Autodesk Inventor part; units mm, degrees
ref_plane "YZ Plane" through (0, 0, 0) normal (1, 0, 0) x (0, 1, 0)
ref_plane "XZ Plane" through (0, 0, 0) normal (0, 1, 0) x (-1, 0, 0)
ref_plane "XY Plane" through (0, 0, 0) normal (0, 0, 1) x (1, 0, 0)
sketch "スケッチ1" plane through (0, 0, 0) normal (0, 0, 1) x (1, 0, 0)
  circle A0 centre (59.9649, 0.0002) radius 1.5
  circle A1 centre (9.9649, 0.0002) radius 2
  circle A2 centre (-5.0351, 0.0002) radius 2
  circle A3 centre (50.4166, -7.2682) radius 1.5
  circle A4 centre (7.9649, -9.9998) radius 1.5
  arc A5 (-5.2274, 4.9965) -> (-7.9614, -4.054) centre (-5.0351, 0.0002) ccw
  line L0 (-7.9614, -4.054) -> (5.3313, -13.6486)
  arc A6 (5.3313, -13.6486) -> (7.4492, -14.4702) centre (7.9649, -9.9998) ccw
  line L1 (7.4492, -14.4702) -> (59.4492, -20.4691)
  arc A7 (59.4492, -20.4691) -> (64.3851, -16.8426) centre (59.9649, -15.9988) ccw
  line L2 (64.3851, -16.8426) -> (67.3319, -1.4061)
  arc A8 (67.3319, -1.4061) -> (59.6765, 7.4946) centre (59.9649, 0.0002) ccw
  line L3 (59.6765, 7.4946) -> (-5.2274, 4.9965)
  circle A9 centre (59.9649, 0.0002) radius 3
  circle A10 centre (50.4166, -7.2682) radius 3
  circle A11 centre (7.9649, -9.9998) radius 3
  circle A12 centre (36.9539, 0.0002) radius 1.5
  circle A13 centre (36.9539, 0.0002) radius 3
  arc A14 (36.6995, 6.6103) -> (33.5984, -5.7005) centre (36.9539, 0.0002) ccw
  line L4 (7.4492, -14.4702) -> (59.4492, -20.4691)
  arc A15 (57.6822, -19.8768) -> (59.4492, -20.4691) centre (59.9649, -15.9988) ccw
  line L5 (33.5984, -5.7005) -> (57.6822, -19.8768)
  line L6 (59.6765, 7.4946) -> (-5.2274, 4.9965)
  point P0 (0, 0)
  point P1 (0, 0)
  dimension "d0" = 6
  dimension "d1" = 6
  dimension "d2" = 6
  dimension "d3" = 6
extrude "押し出し1" add sketch "スケッチ1" along normal blind 3 contours L3 A8 L2 A7 A15 L5 A14 | A9 | A10 | A13
extrude "押し出し2" cut sketch "スケッチ1" along normal blind 1 contours A9 | A10 | A13
sketch "スケッチ2" plane through (0, 0, 0) normal (0, 0, -1) x (-1, 0, 0)
  circle A0 centre (-59.9649, 0.0002) radius 3
  circle A1 centre (-50.4166, -7.2682) radius 3
  circle A2 centre (-36.9539, 0.0002) radius 3
  line L0 (-59.6765, 7.4946) -> (-36.6995, 6.6103)
  arc A3 (-59.6765, 7.4946) -> (-67.3319, -1.4061) centre (-59.9649, 0.0002) ccw
  line L1 (-64.3851, -16.8426) -> (-67.3319, -1.4061)
  arc A4 (-64.3851, -16.8426) -> (-57.6822, -19.8768) centre (-59.9649, -15.9988) ccw
  line L2 (-33.5984, -5.7005) -> (-57.6822, -19.8768)
  arc A5 (-33.5984, -5.7005) -> (-36.6995, 6.6103) centre (-36.9539, 0.0002) ccw
  circle A6 centre (-59.9649, 0.0002) radius 1.5
  circle A7 centre (-50.4166, -7.2682) radius 1.5
  circle A8 centre (-36.9539, 0.0002) radius 1.5
  point P0 (0, 0)
properties part number "ツイン抑え" material "ポリカーボネート、クリア"
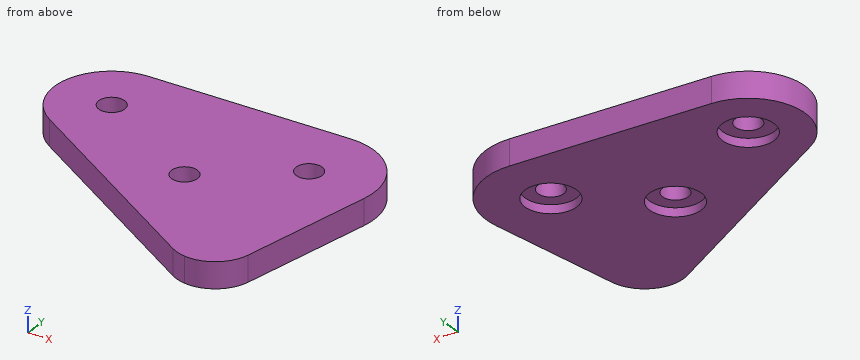
The model under review builds one solid part; all positions refer to its coordinate system, in mm. Coordinates: 2 decimals unless noted, no trailing zeros. Order: outer loops, then holes, each group sorted by start corner. A loop starts at its lowest first (then second) coordinate and runs counter-clockwise, first axis right, second up. Notation, with made-up numbers: M 5,71.25 L 10,71.25 A26 ccw 10,107.25 Z; hole C 64.5,28.25 d4. An arc over 180 degrees is marked long. One line per question, with ' | ' between items.
(1) Add section D-D, the plane y = -5. Write out the cut boundary in (x, z), then the cut area to 3 significant figures.
Geometry results:
outline: M 32.62,0 L 48.45,0 L 48.45,1 L 52.38,1 L 52.38,0 L 66.65,0 L 66.65,3 L 32.62,3 Z | area: 98.1 mm²
(2) Insertion check: pin 1 (4 mm diameter, centred on x = 50.42, y = -7.27, fed in from -Z). The pin has a flat end and moves straight along its axis. Give the tip position at first contact, or say it passes through.
Geometry results:
pin 1: stops at z = 1
(3) Add section A-A, the plane x = 61. Write out the cut boundary in (y, z).
Geometry results:
outline: M -20.38,0 L -2.82,0 L -2.82,1 L -1.09,1 L -1.09,3 L -20.38,3 Z; M 1.09,1 L 2.82,1 L 2.82,0 L 7.43,0 L 7.43,3 L 1.09,3 Z
(4) Add section C-C, the plane z = 1.6. Write out the cut boundary in (x, y).
Geometry results:
outline: M 33.6,-5.7 L 57.68,-19.88 A4.5 ccw 59.45,-20.47 A4.5 ccw 64.39,-16.84 L 67.33,-1.41 A7.5 ccw 59.68,7.49 L 36.7,6.61 A6.61 ccw Z; hole C 36.95,0 d3; hole C 50.42,-7.27 d3; hole C 59.96,0 d3
(5) Add section B-B, the plane y = 0.5. Write out the cut boundary in (x, z).
Geometry results:
outline: M 30.36,0 L 34,0 L 34,1 L 35.54,1 L 35.54,3 L 30.36,3 Z; M 38.37,1 L 39.91,1 L 39.91,0 L 57.01,0 L 57.01,1 L 58.55,1 L 58.55,3 L 38.37,3 Z; M 61.38,1 L 62.92,1 L 62.92,0 L 67.45,0 L 67.45,3 L 61.38,3 Z
(6) For probe 1 along X at (y, z) = (0.25, 2.35); probe 2 along X at (y, z) = (-2, 0.65); probe 3 along Y at (x, z) = (35.5, 0.55), list the stretches that pass through material, from the lowest coordinate up. Write a range as from..to.
Geometry results:
probe 1: x = 30.34..35.47, 38.43..58.49, 61.44..67.46 | probe 2: x = 30.65..34.72, 39.19..57.73, 62.2..67.22 | probe 3: y = -6.82..-2.62, 2.62..6.45
